Solid Edge part; units mm, degrees
sketch "Sketch1" plane through (0, 0, 0) normal (0, 0, 1) x (1, 0, 0)
  circle A0 centre (0, 0) radius 4.25
extrude "Protrusion1" add sketch "Sketch1" along normal blind 5
sketch "Sketch2" plane through (0, 0, 5) normal (0, 0, 1) x (1, 0, 0)
  circle A0 centre (0, 0) radius 2.5
extrude "ExtrudedProtrusion_2" add sketch "Sketch2" along normal blind 15
sketch "Sketch3" plane through (0, 0, 0) normal (0, 0, -1) x (-1, 0, 0)
  line L0 (2.25, 0) -> (1.125, 1.9486)
  line L1 (1.125, 1.9486) -> (-1.125, 1.9486)
  line L2 (-1.125, 1.9486) -> (-2.25, 0)
  line L3 (-2.25, 0) -> (-1.125, -1.9486)
  line L4 (-1.125, -1.9486) -> (1.125, -1.9486)
  line L5 (1.125, -1.9486) -> (2.25, 0)
extrude "ExtrudedCutout_1" cut sketch "Sketch3" against normal blind 2.6
properties material "Stainless steel"
Part model, mm, in its own coordinate system. A direction names the side the tool comes from. Round coordinates to 2 decimals unless told otherwise and drop trailing zeros. Order: outer loops, then holes, each group sorted by start corner. A loop starts at its lowest first (then second) coordinate and runs counter-clockwise, first axis right, second up. Notation, with made-up numbers: M 82.5,85.25 L 105.5,85.25 A25 cw 105.5,117.25 Z; hole C 16,58 d10. An arc over 180 degrees is marked long. Answer in a Markdown table with one row per item. Add a question column.
Q1. Cut at B-B on y = 0.75. Give the cut face in (x, z), and give its area (3 significant figures).
Q2. Mould opens along Y. For faces 4 (the face through (2, -1, 0)), 5 (the face through (2.285, -3.584, 2.465)), 6 (the face through (-1.68, -0.99, 1.28)), 7 (the face through (-1.695, 0.961, 1.282)) say: +Y half, -Y half, draft (parallel to the pull), parting line (faces both ways), or undercut.
Q3. Wall check: L1, parallel to Z at x = -1, y = 0.75; L2, parallel to Z at x = -1.5, y = -2.25; L3, parallel to X at y = -2.25, z = 4.75. Give the ranges that are in metal, low to high. Write a range as from..to.
Q4. 3-axis set-ups, long thin cutter, end or side, ignore diameter. For faces 1 (the face through (0, 0, 20)), 2 (the face through (1.695, -0.961, 1.282)), 3 (the face through (-0.54, 2.44, 12.4)): which of +Z, -Z, +X, -X, +Y, -Y reach the whole face in a straight line?
Q5. Cut at D-D on y = -3. Give the cut face in (x, z), and give its area (3 significant figures).
Q6. Pin check, flat tips, straight feed: pin 1 (3 mm diameter, centred on y = -1.5, z = 16, fed in from -X); pin 2 (1 mm diameter, centred on y = -2, z = 9.5, fed in from +X); pin 3 (4 mm diameter, centred on y = -2.5, z = 15.5, fed in from -X); pin 4 (1.8 mm diameter, centred on x = 0.5, z = 2, fed in from +Y). Stop position of each tip, or through.
Q7. Cut at A-A on x = 0. Give the cut face in (y, z).
Q8. Cut at C-C on z = 18.5. Give the cut face in (x, y).
Established:
| question | item | result |
|---|---|---|
| 1 | outline | M -4.18,0 L -1.82,0 L -1.82,2.6 L 1.82,2.6 L 1.82,0 L 4.18,0 L 4.18,5 L 2.38,5 L 2.38,20 L -2.38,20 L -2.38,5 L -4.18,5 Z |
| 1 | area | 104 mm2 |
| 2 | face 4 | draft |
| 2 | face 5 | parting line |
| 2 | face 6 | undercut |
| 2 | face 7 | undercut |
| 3 | L1 | z = 2.6..20 |
| 3 | L2 | z = 0..5 |
| 3 | L3 | x = -3.61..3.61 |
| 4 | face 1 | +Z, +X, -X, +Y, -Y |
| 4 | face 2 | -Z |
| 4 | face 3 | +Z |
| 5 | outline | M -3.01,0 L 3.01,0 L 3.01,5 L -3.01,5 Z |
| 5 | area | 30.1 mm2 |
| 6 | pin 1 | stops at x = -2.5 |
| 6 | pin 2 | stops at x = 2 |
| 6 | pin 3 | stops at x = -2.45 |
| 6 | pin 4 | stops at y = 4.25 |
| 7 | outline | M -4.25,0 L -1.95,0 L -1.95,2.6 L 1.95,2.6 L 1.95,0 L 4.25,0 L 4.25,5 L 2.5,5 L 2.5,20 L -2.5,20 L -2.5,5 L -4.25,5 Z |
| 8 | outline | C 0,0 d5 |
